Could you check a few things on this model? Use its own coordinates, in mm. A direction names the side the tool comes from. Give positions to 0.01 mm unless a question says otherwise; leave off trailing zeros. Write each loop counter-clockwise with the first axis right and the second up, starting at its lowest first coordinate (ties: lowest second). Pieces come first, ordered by that corner, then holes. Notation, with made-up numbers: M -6.75,78.25 L 50.25,78.25 A18 cw 50.25,98.25 Z; hole C 22,-39.75 d8. An arc over 180 degrees is marked long. Answer as a JSON object with one key per item and string values. Group by question number.
```python
from build123d import *

# Parameters (mm, degrees)
SKETCH1_W           = 152.4
SKETCH1_H           = 88.9
BOSS_EXTRUDE1_DEPTH = 2.54
SKETCH2_W           = 2.54
SKETCH2_H           = 63.5
SKETCH2_W_2         = 114.3
SKETCH2_H_2         = 2.54
BOSS_EXTRUDE2_DEPTH = 3.175
FILLET1_R           = 2.54
SKETCH3_R           = 3.49631
SKETCH3_R_2         = 2.794
CUT_EXTRUDE1_DEPTH  = 2.54
SKETCH5_R           = 2.286
CUT_EXTRUDE2_DEPTH  = 89.401944125
SKETCH7_R           = 50.8
BOSS_EXTRUDE3_DEPTH = 2.54
SKETCH8_R           = 3.556
CUT_EXTRUDE3_DEPTH  = 103.722904092


with BuildPart() as part:
    # Sketch1 → Boss-Extrude1 (new body)
    with BuildSketch(Plane(origin=(0, 0, 0), x_dir=(1, 0, 0), z_dir=(0, 1, 0))):
        Rectangle(SKETCH1_W, SKETCH1_H)
    extrude(amount=BOSS_EXTRUDE1_DEPTH)

    # Sketch2 → Boss-Extrude2 (add)
    with BuildSketch(Plane.XZ):
        with Locations((-72.39, 0)):
            Rectangle(SKETCH2_W, SKETCH2_H)
        with Locations((72.39, 0)):
            Rectangle(SKETCH2_W, SKETCH2_H)
        with Locations((0, 40.64)):
            Rectangle(SKETCH2_W_2, SKETCH2_H_2)
        with Locations((0, -40.64)):
            Rectangle(SKETCH2_W_2, SKETCH2_H_2)
    extrude(amount=BOSS_EXTRUDE2_DEPTH)

    # Fillet1
    fillet1_edges = [part.edges().sort_by_distance(p)[0] for p in [
        (76.2, 1.27, 44.45),
        (-76.2, 1.27, 44.45),
        (-76.2, 1.27, -44.45),
        (76.2, 1.27, -44.45),
    ]]
    fillet(fillet1_edges, radius=FILLET1_R)

    # Sketch3 → Cut-Extrude1 (cut)
    with BuildSketch(Plane(origin=(0, 2.54, 0), x_dir=(1, 0, 0), z_dir=(0, 1, 0))):
        with Locations(Location((38.1, 0, 0), (0, 0, 270))):
            Circle(SKETCH3_R)
        with Locations(Location((-25.4, 0, 0), (0, 0, 270))):
            Circle(SKETCH3_R_2)
    extrude(amount=-CUT_EXTRUDE1_DEPTH, mode=Mode.SUBTRACT)

    # Sketch5 → Cut-Extrude2 (cut, through all)
    with BuildSketch(Plane(origin=(0, 2.54, 0), x_dir=(1, 0, 0), z_dir=(0, 1, 0))):
        with Locations(Location((-50.8, 12.7, 0), (0, 0, 270))):
            Circle(SKETCH5_R)
        with Locations(Location((-50.8, -12.7, 0), (0, 0, 90))):
            Circle(SKETCH5_R)
    extrude(amount=-CUT_EXTRUDE2_DEPTH, mode=Mode.SUBTRACT)

    # Sketch7 → Boss-Extrude3 (add)
    with BuildSketch(Plane(origin=(0, 2.54, 0), x_dir=(1, 0, 0), z_dir=(0, 1, 0))):
        with Locations(Location((38.1, 0, 0), (0, 0, 61.044975628))):
            Circle(SKETCH7_R)
    extrude(amount=BOSS_EXTRUDE3_DEPTH)

    # Sketch8 → Cut-Extrude3 (cut, through all)
    with BuildSketch(Plane(origin=(0, 5.08, 0), x_dir=(1, 0, 0), z_dir=(0, 1, 0))):
        with Locations(Location((38.1, 0, 0), (0, 0, 270))):
            Circle(SKETCH8_R)
    extrude(amount=-CUT_EXTRUDE3_DEPTH, mode=Mode.SUBTRACT)


solid = part.part
```
1) I'm going to push flat-ended pins straight in: pin 1 (10 mm diameter, centred on x = 84.5, z = -16, fed in from -Y); pin 2 (6 mm diameter, centred on x = -50.8, z = -12.7, fed in from -Y); pin 3 (4 mm diameter, centred on y = -2.5, z = -31.5, fed in from -X); pin 4 (2 mm diameter, centred on y = -1.5, z = 36.5, fed in from +X). Where does each tip first touch, or does it pass through?
2) If we section it at C-C, the plane y = -1.5: List the corners of the cut face in (x, z) for me.
3) For faces 4 (the flat face through (-1, -2, 41.91)), 5 (the flat face through (71.12, -2, 0)), 6 (the flat face through (72, 2.54, 41)), which set-ups out of +Z, -Z, +X, -X, +Y, -Y let a thin tool reach every point of the face, with its end or its side?
4) If we section it at D-D, the plane x = -25.4: List the corners of the cut face in (y, z) for me (3 decimals), plus the area to 3 significant figures.
5) Please list where these lines run through material, in increasing order: line 1 along X through (y, z) = (2.05, 0); line 2 along X through (y, z) = (-2.25, 1.5); line 3 along X through (y, z) = (1.6, 12.7). Write a range as from..to.
6) We'd pull the mould along X, two halves only. Please class faces 1 (the flat face through (-73.66, -2, 0)), 2 (the flat face through (37, 2.54, -47)), 3 (the cylindrical face through (-28.128, 1.288, -0.606)): released by +X, released by -X, zero draft, split by the parting line, or undercut.
7) If we section it at A-A, the plane x = 38.1: List the corners of the cut face in (y, z) for me (3 decimals).
8) If we section it at B-B, the plane z = 0: List the corners of the cut face in (x, y) for me (3 decimals).
Taken from the geometry:
{
 "1": {"pin 1": "y = 2.54", "pin 2": "y = 0", "pin 3": "x = -73.66", "pin 4": "through"},
 "2": {"outline": "M -73.66,-31.75 L -71.12,-31.75 L -71.12,31.75 L -73.66,31.75 Z; M -57.15,-41.91 L 57.15,-41.91 L 57.15,-39.37 L -57.15,-39.37 Z; M -57.15,39.37 L 57.15,39.37 L 57.15,41.91 L -57.15,41.91 Z; M 71.12,-31.75 L 73.66,-31.75 L 73.66,31.75 L 71.12,31.75 Z"},
 "3": {"face 4": "+Z, +X, -X, -Y", "face 5": "+Z, -Z, -Y", "face 6": "+Z, +X, +Y"},
 "4": {"outline": "M -3.175,-41.91 L 0,-41.91 L 0,-44.45 L 2.54,-44.45 L 2.54,-2.794 L 0,-2.794 L 0,-39.37 L -3.175,-39.37 Z; M -3.175,39.37 L 0,39.37 L 0,2.794 L 2.54,2.794 L 2.54,44.45 L 0,44.45 L 0,41.91 L -3.175,41.91 Z", "area": "228 mm²"},
 "5": {"line 1": "-76.2..-28.19, -22.61..34.54, 41.66..76.2", "line 2": "-73.66..-71.12, 71.12..73.66", "line 3": "-76.2..-53.09, -48.51..76.2"},
 "6": {"face 1": "released by -X", "face 2": "zero draft", "face 3": "undercut"},
 "7": {"outline": "M -3.175,-41.91 L 0,-41.91 L 0,-44.45 L 2.54,-44.45 L 2.54,-50.8 L 5.08,-50.8 L 5.08,-3.556 L 0,-3.556 L 0,-39.37 L -3.175,-39.37 Z; M -3.175,39.37 L 0,39.37 L 0,3.556 L 5.08,3.556 L 5.08,50.8 L 2.54,50.8 L 2.54,44.45 L 0,44.45 L 0,41.91 L -3.175,41.91 Z"},
 "8": {"outline": "M -76.2,0 L -73.66,0 L -73.66,-3.175 L -71.12,-3.175 L -71.12,0 L -28.194,0 L -28.194,2.54 L -76.2,2.54 Z; M -22.606,0 L 34.544,0 L 34.544,5.08 L -12.7,5.08 L -12.7,2.54 L -22.606,2.54 Z; M 41.656,0 L 71.12,0 L 71.12,-3.175 L 73.66,-3.175 L 73.66,0 L 76.2,0 L 76.2,2.54 L 88.9,2.54 L 88.9,5.08 L 41.656,5.08 Z"}
}
